```python
from build123d import *

# Parameters (mm, degrees)
EXTRUDE_1_DEPTH      = 54.5
EXTRUDE_1_DEPTH_BACK = 49.5
SKETCH_4_R           = 2.25
CUT_EXTRUDE_1_DEPTH  = 111.354474309
SKETCH_5_R           = 4.25
CUT_EXTRUDE_2_DEPTH  = 4
SKETCH_6_R           = 2.75
CUT_EXTRUDE_3_DEPTH  = 89.184465752
CHAMFER_1_SIZE       = 2.5
CUT_EXTRUDE_4_DEPTH  = 89.184465752
SKETCH_10_W          = 20
SKETCH_10_H          = 4.7
EXTRUDE_2_DEPTH      = 10
FILLET_1_R           = 5


with BuildPart() as part:
    # ｽｹｯﾁ3 → ﾎﾞｽ - 押し出し1 (new, two sides: drawn at the far end of the back side and taken through both)
    with BuildSketch(Plane.XY.offset(-EXTRUDE_1_DEPTH_BACK)):
        Polygon((-57.5, 8.1), (-49.5, 8.1), (-49.5, -21.9), (41, -21.9), (41, -31.9), (-62.5, -31.9), (-62.5, -21.9), (-57.5, -21.9), align=None)
    extrude(amount=EXTRUDE_1_DEPTH + EXTRUDE_1_DEPTH_BACK)

    # ｽｹｯﾁ4 → ｶｯﾄ - 押し出し1 (cut, through all)
    with BuildSketch(Plane(origin=(-49.5, 0, 0), x_dir=(0, 0, -1), z_dir=(1, 0, 0))):
        with Locations(Location((-39.5, -6.9, 0), (0, 0, 90))):
            Circle(SKETCH_4_R)
        with Locations(Location((39.5, -6.9, 0), (0, 0, 90))):
            Circle(SKETCH_4_R)
    extrude(amount=-CUT_EXTRUDE_1_DEPTH, mode=Mode.SUBTRACT)

    # ｽｹｯﾁ5 → ｶｯﾄ - 押し出し2 (cut)
    with BuildSketch(Plane(origin=(-49.5, 0, 0), x_dir=(0, 0, -1), z_dir=(1, 0, 0))):
        with Locations(Location((-39.5, -6.9, 0), (0, 0, 90))):
            Circle(SKETCH_5_R)
        with Locations(Location((39.5, -6.9, 0), (0, 0, 90))):
            Circle(SKETCH_5_R)
    extrude(amount=-CUT_EXTRUDE_2_DEPTH, mode=Mode.SUBTRACT)

    # ｽｹｯﾁ6 → ｶｯﾄ - 押し出し3 (cut, through all)
    with BuildSketch(Plane(origin=(0, -21.9, 0), x_dir=(1, 0, 0), z_dir=(0, 1, 0))):
        with Locations(Location((-39.485, 32.4, 0), (0, 0, 270))):
            Circle(SKETCH_6_R)
        with Locations(Location((31.485, 32.4, 0), (0, 0, 270))):
            Circle(SKETCH_6_R)
        with Locations(Location((31.485, -32.4, 0), (0, 0, 270))):
            Circle(SKETCH_6_R)
        with Locations(Location((-39.485, -32.4, 0), (0, 0, 270))):
            Circle(SKETCH_6_R)
    extrude(amount=-CUT_EXTRUDE_3_DEPTH, mode=Mode.SUBTRACT)

    # 面取り1
    chamfer_1_edges = [part.edges().sort_by_distance(p)[0] for p in [
        (-39.485, -21.9, -35.15),
        (31.485, -21.9, -35.15),
        (31.485, -21.9, 29.65),
        (-39.485, -21.9, 29.65),
    ]]
    chamfer(chamfer_1_edges, length=CHAMFER_1_SIZE)

    # ｽｹｯﾁ7 → ｶｯﾄ - 押し出し4 (cut, through all)
    with BuildSketch(Plane(origin=(0, -21.9, 0), x_dir=(1, 0, 0), z_dir=(0, 1, 0))):
        with BuildLine():
            ThreePointArc((22.203162897, -44.5), (16.96784035, -27.729392364), (31, -17.157714246))
            Line((31, -17.157714246), (31, 17.157714246))
            ThreePointArc((31, 17.157714246), (18.30682719, 24.725479729), (17.988611594, 39.5))
            Line((17.988611594, 39.5), (-25.988611594, 39.5))
            ThreePointArc((-25.988611594, 39.5), (-24.679892382, 36.056677236), (-24.235, 32.4))
            ThreePointArc((-24.235, 32.4), (-28.706926192, 21.611319589), (-39.5, 17.150007377))
            Line((-39.5, 17.150007377), (-39.5, -17.150007377))
            ThreePointArc((-39.5, -17.150007377), (-28.706926192, -21.611319589), (-24.235, -32.4))
            ThreePointArc((-24.235, -32.4), (-25.808185389, -39.14590558), (-30.203162897, -44.5))
            Line((-30.203162897, -44.5), (22.203162897, -44.5))
        make_face()
    extrude(amount=-CUT_EXTRUDE_4_DEPTH, mode=Mode.SUBTRACT)

    # ｽｹｯﾁ10 → ﾎﾞｽ - 押し出し2 (add)
    with BuildSketch(Plane(origin=(0, -21.9, 0), x_dir=(1, 0, 0), z_dir=(0, 1, 0))):
        with Locations((-39.5, -52.15)):
            Rectangle(SKETCH_10_W, SKETCH_10_H)
        with Locations((31, -52.15)):
            Rectangle(SKETCH_10_W, SKETCH_10_H)
    extrude(amount=EXTRUDE_2_DEPTH)

    # ﾌｨﾚｯﾄ1
    fillet_1_edges = [part.edges().sort_by_distance(p)[0] for p in [
        (-62.5, -26.9, -49.5),
        (31, -26.9, 17.157714246),
        (22.203162897, -26.9, 44.5),
        (-30.203162897, -26.9, 44.5),
        (-39.5, -26.9, 17.150007377),
        (-39.5, -26.9, -17.150007377),
        (-25.988611594, -26.9, -39.5),
        (17.988611594, -26.9, -39.5),
        (31, -26.9, -17.157714246),
        (-29.5, -11.9, 52.15),
        (21, -11.9, 52.15),
        (41, -26.9, -49.5),
        (-62.5, -26.9, 54.5),
        (41, -21.9, 54.5),
        (-53.5, 8.1, 54.5),
        (-53.5, 8.1, -49.5),
    ]]
    fillet(fillet_1_edges, radius=FILLET_1_R)


solid = part.part
```
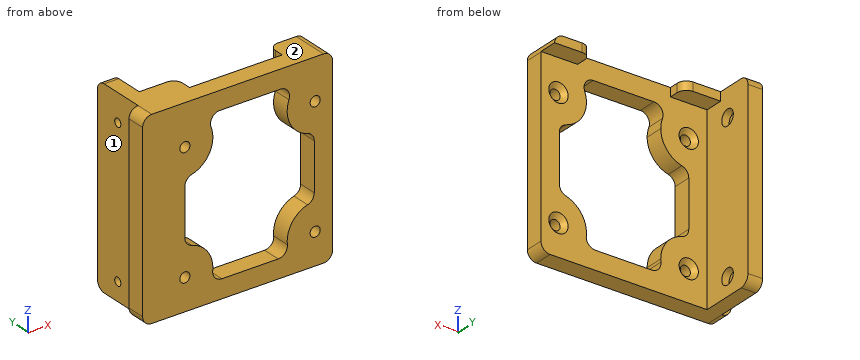
Geometry: final body of the model. Coordinates: model frame, mm. Face numbers are marked on the shaded views. A direction names the side the tool comes from. Round coordinates to 2 decimals unless told otherwise and drop trailing zeros. Order: outer loops, then holes, each group sorted by start corner. A loop starts at its lowest first (then second) coordinate and runs counter-clockwise, first axis right, second up. Notation, with made-up numbers: (68, -9) - (109, -9) arc R33 ccw to (109, 23) - close; hole circle Ø10 at (-0.75, -26). An arc over 180 degrees is marked (long way). Write item = value, one per line. Start each with the question number.
Q1. Pin query (flat end, axial travel): pin 1 (8 mm diameter, centred on x = -40, y = -16.5, fed in from -Z); pin 2 (24 mm diameter, centred on y = -0.5, z = -3, fed in from -X); pin 3 (6 mm diameter, centred on y = -19.5, z = -20.5, fed in from +X); pin 4 (5 mm diameter, centred on x = -44.5, z = 53, fed in from +Y). Return the tip coordinate at first contact, or that it passes through.
Q2. Access query for the marked faces 1 and 2. Directions: +Z, -Z, +X, -X, +Y, -Y. A direction counts if a zero-diameter tool reaches every point of the face in a straight line with its end or side. Return the directions, or none.
Q3. Cut plane A-A on x = -3.5. Return the cut outline in (y, z).
Q4. Cut plane B-B on y = -6.9. Return the cut outline in (x, z).
Q5. Ray query, line 1 (Z direction, x = -51, y = -7); line 2 (Y direction, x = -52, z = -39); line 3 (X direction, y = -24, z = 39). Return the intervals inside material, ascending. Write a range as from..to.
Q6. Cut plane C-C on z = -20.5. Return the cut outline in (x, y), and give its area (3 significant figures).
Q7. Cut plane D-D on y = -19.5. Return the cut outline in (x, z).
Outcome:
q1.pin_1 = 49.8
q1.pin_2 = -57.5
q1.pin_3 = 41
q1.pin_4 = -11.9
q2.face_1 = +Z, -Z, -X, +Y
q2.face_2 = +Z, +X, -X, +Y, -Y
q3.outline = (-31.9, -49.5) - (-21.9, -49.5) - (-21.9, -39.5) - (-31.9, -39.5) - close; (-31.9, 44.5) - (-21.9, 44.5) - (-21.9, 54.5) - (-31.9, 54.5) - close
q4.outline = (-57.5, -49.5) - (-49.5, -49.5) - (-49.5, -43.75) - (-53.5, -43.75) - (-53.5, -41.75) - (-57.5, -41.75) - close; (-57.5, -37.25) - (-53.5, -37.25) - (-53.5, -35.25) - (-49.5, -35.25) - (-49.5, 35.25) - (-53.5, 35.25) - (-53.5, 37.25) - (-57.5, 37.25) - close; (-57.5, 41.75) - (-53.5, 41.75) - (-53.5, 43.75) - (-49.5, 43.75) - (-49.5, 54.5) - (-57.5, 54.5) - close
q5.line_1 = -49.5..-43.75, -35.25..35.25, 43.75..54.5
q5.line_2 = -31.9..-11.12, -2.68..8.1
q5.line_3 = -62.5..-25.5, 17.5..41
q6.outline = (-62.5, -31.9) - (-29.95, -31.9) - (-29.95, -21.9) - (-49.5, -21.9) - (-49.5, 8.1) - (-57.5, 8.1) - (-57.5, -21.9) - (-62.5, -21.9) - close; (21.95, -31.9) - (41, -31.9) - (41, -21.9) - (21.95, -21.9) - close
q6.area = 756 mm^2
q7.outline = (-57.5, -49.5) - (-49.5, -49.5) - (-49.5, 49.8) - (-29.5, 49.8) - (-29.5, 54.5) - (-57.5, 54.5) - close; (21, 49.8) - (40.99, 49.8) arc R5 ccw to (36, 54.5) - (21, 54.5) - close
